Verification items for the finished model (mm, model axes). Face numbers are marked on the shaded views. Round coordinates to 2 decimals unless told otherwise and drop trailing zeros. Order: outer loops, then holes, each group sorted by start corner. A loop starts at its lowest first (then second) coordinate and runs counter-clockwise, first axis right, second up. Notation, with made-up numbers: (-36, 63) -> (4, 63) arc R20 cw to (4, 68) -> close; hole circle Ø5 at (-14.5, 50). An arc over 180 degrees is marked (long way). Answer in a Markdown table with one row per item. Add a question column.
```python
from build123d import *

# Parameters (mm, degrees)
SKETCH_1_W      = 100
SKETCH_1_H      = 34
SKETCH_1_R      = 10
EXTRUDE_1_DEPTH = 5
SKETCH_1_2_R    = 10
EXTRUDE_2_DEPTH = 10


with BuildPart() as part:
    # Sketch 1 → Extrude 1 (new body)
    with BuildSketch(Plane(origin=(0, 0, 0), x_dir=(1, 0, 0), z_dir=(0, 1, 0))):
        Rectangle(SKETCH_1_W, SKETCH_1_H)
        with Locations(Location((0, 0, 0), (0, 0, 270))):
            Circle(SKETCH_1_R, mode=Mode.SUBTRACT)
        Polygon((-40, 10), (-20, 10), (-25, 0), (-20, -10), (-40, -10), (-35, 0), align=None, mode=Mode.SUBTRACT)
        Polygon((40, 10), (20, 10), (25, 0), (20, -10), (40, -10), (35, 0), align=None, mode=Mode.SUBTRACT)
    extrude(amount=EXTRUDE_1_DEPTH)

    # Sketch 1_2 → Extrude 2 (add)
    with BuildSketch(Plane(origin=(0, 0, 0), x_dir=(1, 0, 0), z_dir=(0, 1, 0))):
        Polygon((-40, -10), (-20, -10), (-25, 0), (-20, 10), (-40, 10), (-35, 0), align=None)
        with Locations(Location((0, 0, 0), (0, 0, 270))):
            Circle(SKETCH_1_2_R)
        Polygon((40, -10), (20, -10), (25, 0), (20, 10), (40, 10), (35, 0), align=None)
    extrude(amount=EXTRUDE_2_DEPTH)


solid = part.part
```
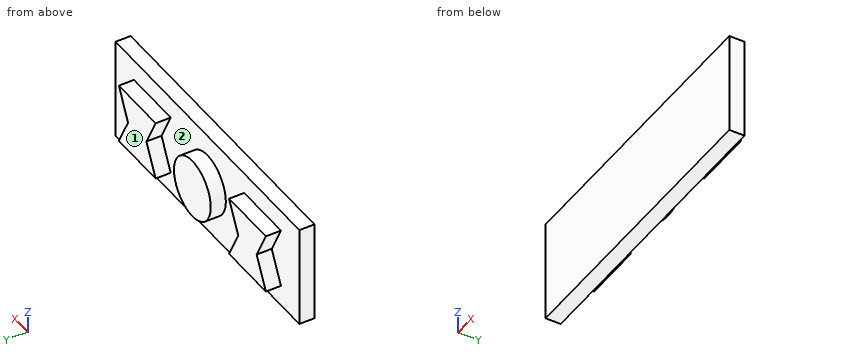
1) Depth check by flat-ended pin: P1, Ø5.5, axis at x = 31, y = 8, coming from the -Z side; P2, Ø3, axis at x = -8, z = 11, coming from the +Y side. Enter the tip coordinate at first touch or a pass-through.
2) Cross-section at C-C, the plane z = -4. Record the boundary of the cut face in (x, y).
3) Cross-section at A-A, the plane y = 6. Record the boundary of the cut face in (x, z).
4) Cross-section at D-D, the plane x = 23.5. Record the boundary of the cut face in (y, z), and give its area (3 significant figures).
5) Cross-section at B-B, the plane x = 0. Record the boundary of the cut face in (y, z).
6) Thickness scan on L1, parallel to X at y = 8.75, z = -5; L2, parallel to X at y = 6.5, z = -1; L3, parallel to Y at x = -17, z = -13.5. Record the ranges inside material, lowest first. Write a range as [from, to].
7) Draft check along X on the marked faces 1 and 2. Enter one of: +X half, -X half, draft (parallel to the pull), parting line (faces both ways), or undercut.
Results below:
| question | item | result |
|---|---|---|
| 1 | P1 | z = -10 |
| 1 | P2 | y = 5 |
| 2 | outline | (-50, 0) -> (50, 0) -> (50, 5) -> (37, 5) -> (37, 10) -> (23, 10) -> (23, 5) -> (9.17, 5) -> (9.17, 10) -> (-9.17, 10) -> (-9.17, 5) -> (-23, 5) -> (-23, 10) -> (-37, 10) -> (-37, 5) -> (-50, 5) -> close |
| 3 | outline | (-40, -10) -> (-20, -10) -> (-25, 0) -> (-20, 10) -> (-40, 10) -> (-35, 0) -> close; circle Ø20 at (0, 0); (20, -10) -> (40, -10) -> (35, 0) -> (40, 10) -> (20, 10) -> (25, 0) -> close |
| 4 | outline | (0, -17) -> (5, -17) -> (5, -10) -> (10, -10) -> (10, -3) -> (5, -3) -> (5, 3) -> (10, 3) -> (10, 10) -> (5, 10) -> (5, 17) -> (0, 17) -> close |
| 4 | area | 240 mm² |
| 5 | outline | (0, -17) -> (5, -17) -> (5, -10) -> (10, -10) -> (10, 10) -> (5, 10) -> (5, 17) -> (0, 17) -> close |
| 6 | L1 | [-37.5, -22.5], [-8.66, 8.66], [22.5, 37.5] |
| 6 | L2 | [-35.5, -24.5], [-9.95, 9.95], [24.5, 35.5] |
| 6 | L3 | [0, 5] |
| 7 | face 1 | draft |
| 7 | face 2 | undercut |
